Job drawing, mm, ordinate dimensions from the low corner. One solid piece. Give positions to 0.01 mm unless a question says otherwise; leave off trailing zeros. Write each loop counter-clockwise with the first axis right and the second up, starting at its lowest first coordinate (ties: lowest second). Pieces come first, ordered by that corner, then holes. Notation, with made-up numbers: M -0.75,-14 L 41.25,-14 A15 ccw 41.25,3 Z; hole C 30.5,79.25 d3. An arc over 180 degrees is marked long. Answer as CSV lines item,"result". Start each with the question number.
1) Slice it at A-A, the plane z = 2.15. Give the cut face in (x, y).
2) Mould opens along X. For the marked faces 1, 2, 3 and 4 say: pulls with the +X half, pulls with the -X half, needs draft (parallel to the pull), parting line crosses it, or undercut.
3) Slice it at D-D, the plane x = 2.65. Give the cut face in (y, z) (1 decimal).
4) Slice it at C-C, the plane z = 0.25. Give the cut face in (x, y).
5) Slice it at B-B, the plane y = 6.25. Give the cut face in (x, z), plus the area to 3 significant figures.
6) Wall check: line 1 along X through (y, z) = (9.5, 2.1) (1 decimal); line 2 along X through (y, z) = (10.5, 2.55) (1 decimal); line 3 along Z through (x, y) = (3.5, 10). Give the ranges that are in metal, low to high. Write a range as from..to.
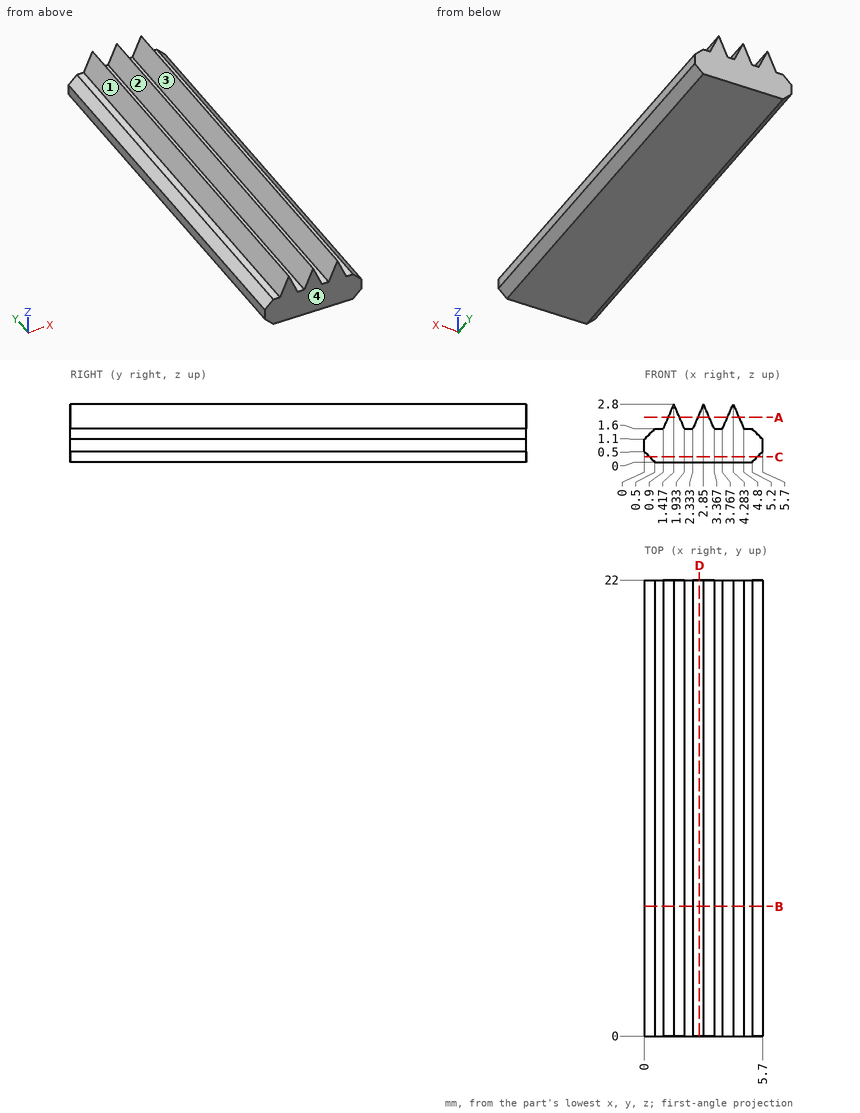
Found:
1,outline,"M 1.14,0 L 1.7,0 L 1.7,22 L 1.14,22 Z; M 2.57,0 L 3.13,0 L 3.13,22 L 2.57,22 Z; M 4,0 L 4.56,0 L 4.56,22 L 4,22 Z"
2,face 1,"pulls with the -X half"
2,face 2,"undercut"
2,face 3,"undercut"
2,face 4,"needs draft"
3,outline,"M 0,0 L 22,0 L 22,2.3 L 0,2.3 Z"
4,outline,"M 0.25,0 L 5.45,0 L 5.45,22 L 0.25,22 Z"
5,outline,"M 0,0.5 L 0.5,0 L 5.2,0 L 5.7,0.5 L 5.7,1.1 L 5.2,1.6 L 4.8,1.6 L 4.28,2.8 L 3.77,1.6 L 3.37,1.6 L 2.85,2.8 L 2.33,1.6 L 1.93,1.6 L 1.42,2.8 L 0.9,1.6 L 0.5,1.6 L 0,1.1 Z"
5,area,"10.5 mm²"
6,line 1,"1.1..1.7, 2.5..3.2, 4..4.6"
6,line 2,"1.3..1.5, 2.7..3, 4.2..4.4"
6,line 3,"0..1.6"
